CAD build for the part. Positions are in the model's coordinates, mm. A direction names the side the tool comes from. Round coordinates to 2 decimals unless told otherwise and drop trailing zeros. Order: outer loops, then holes, each group sorted by start corner. A loop starts at its lowest first (then second) coordinate and runs counter-clockwise, first axis right, second up. Notation, with made-up numbers: (38, 40.25) - (89, 40.25) arc R20 cw to (89, 50.25) - close; hole circle Ø10 at (-32.75, 27.25). An arc over 180 degrees is marked (long way). Write item = value, one per line.
from build123d import *

# Parameters (mm, degrees)
F1_DEPTH = 40
F2_R     = 5
F3_R     = 2.15
F4_DEPTH = 25
F5_W     = 4.5
F5_H     = 10
F6_DEPTH = 53.001
F7_R     = 2.24999


# Not quite as in the source:
# - a fillet or chamfer is up to 0.001 mm smaller than in the source, because OpenCascade refuses the exact size


with BuildPart() as f1:
    # F0 (on Front) → F1 (new body)
    with BuildSketch(Plane.XZ):
        Polygon((22.5, -17), (26.5, -17), (26.5, 17), (-26.5, 17), (-26.5, -17), (-22.5, -17), (-22.5, 13), (22.5, 13), align=None)
    extrude(amount=F1_DEPTH)

    # F2
    f2_edges = [f1.edges().sort_by_distance(p)[0] for p in [
        (-26.5, -20, 17),
        (26.5, -20, 17),
    ]]
    fillet(f2_edges, radius=F2_R)

    # F3 (on face) → F4 (cut)
    with BuildSketch(Plane.XY.offset(17)):
        with Locations((0, -20)):
            Circle(F3_R)
    extrude(amount=-F4_DEPTH, mode=Mode.SUBTRACT)

    # F5 (on face) → F6 (cut, through all)
    with BuildSketch(Plane.YZ.offset(26.5)):
        with Locations((-20, -7.5)):
            Rectangle(F5_W, F5_H)
    extrude(amount=-F6_DEPTH, mode=Mode.SUBTRACT)

    # F7 (radius 2.25 in the source; OpenCascade refuses exactly that, so slightly less here)
    f7_edges = [f1.edges().sort_by_distance(p)[0] for p in [
        (24.5, -17.75, -2.5),
        (24.5, -22.25, -2.5),
        (24.5, -17.75, -12.5),
        (24.5, -22.25, -12.5),
        (-24.5, -17.75, -2.5),
        (-24.5, -17.75, -12.5),
        (-24.5, -22.25, -2.5),
        (-24.5, -22.25, -12.5),
    ]]
    fillet(f7_edges, radius=F7_R)


solid = f1.part
(1) Band-saw the part on D-D on y = -19. List the corners of the cut face in (x, z), plus the area to 3 significant figures.
Solved:
outline = (-26.5, -17) - (-22.5, -17) - (-22.5, -12.27) - (-26.5, -12.27) - close; (-26.5, -2.73) - (-22.5, -2.73) - (-22.5, 13) - (-1.9, 13) - (-1.9, 17) - (-21.5, 17) arc R5 ccw to (-26.5, 12) - close; (1.9, 13) - (22.5, 13) - (22.5, -2.73) - (26.5, -2.73) - (26.5, 12) arc R5 ccw to (21.5, 17) - (1.9, 17) - close; (22.5, -17) - (26.5, -17) - (26.5, -12.27) - (22.5, -12.27) - close
area = 350 mm²
(2) Probe line 1 along X through (y, z) = (-6, 9.5); line 2 along Y through (x, z) = (0, 14); line 3 along Z through (x, y) = (12.5, -7). List the from-to ranges inside material, lowest first.
Solved:
line_1 = -26.5 to -22.5, 22.5 to 26.5
line_2 = -40 to -22.15, -17.85 to 0
line_3 = 13 to 17
(3) Band-saw the part on C-C on y = -27. List the corners of the cut face in (x, z), plus the area to 3 significant figures.
Solved:
outline = (-26.5, -17) - (-22.5, -17) - (-22.5, 13) - (22.5, 13) - (22.5, -17) - (26.5, -17) - (26.5, 12) arc R5 ccw to (21.5, 17) - (-21.5, 17) arc R5 ccw to (-26.5, 12) - close
area = 441 mm²
(4) Drop flat-ended pins along their axis: pin 1 (6 mm diameter, centred on x = -18.5, y = -17, fed in from -Z); pin 2 (7 mm diameter, centred on x = 0, y = -20, fed in from +Z). Give the stop position or say it passes through.
Solved:
pin_1 = 13
pin_2 = 17
(5) Band-saw the part on A-A on z = 11. List the corners of the cut face in (x, y).
Solved:
outline = (-26.5, -40) - (-22.5, -40) - (-22.5, 0) - (-26.5, 0) - close; (22.5, -40) - (26.5, -40) - (26.5, 0) - (22.5, 0) - close
(6) Tool access for faces 1 (the flat face through (26.5, -20, 1)), 2 (the flat face through (0, -24, 13)), 3 (the flat face through (-24, -17.75, -8)): list every direction of +Z, -Z, +X, -X, +Y, -Y with a clear straight run to the whole face (end or side of a thin tool).
Solved:
face_1 = +Z, -Z, +X, +Y, -Y
face_2 = -Z, +Y, -Y
face_3 = +X, -X
(7) Band-saw the part on B-B on x = 0. List the corners of the cut face in (y, z), plus the area to 3 significant figures.
Solved:
outline = (-40, 13) - (-22.15, 13) - (-22.15, 17) - (-40, 17) - close; (-17.85, 13) - (0, 13) - (0, 17) - (-17.85, 17) - close
area = 143 mm²
(8) Pull direction Z, two halves, no side cores. Call faces 4 (the cylindrical face through (24.47, -18.43, -3.14)), 5 (the cylindrical face through (-0.47, -22.1, 15.03)), 6 (the flat face through (-24, -22.25, -8)), 7 (the cylindrical face through (25.07, -20.28, 15.5)): released by +Z, released by -Z, zero draft, split by the parting line, or undercut.
Solved:
face_4 = undercut
face_5 = zero draft
face_6 = undercut
face_7 = released by +Z
